Can you work these out from the model? Positions are in its coordinate system, mm. Give positions to 0.01 mm unless a question says otherwise; leave off trailing zeros. Use one line per item in the form item = value. Start each with the question number.
1) We'd pull the mould along X, two halves only. Please class faces 1 (the flat face through (0, 0, 12.326)), 2 (the cylindrical face through (-1.924, 0.028, -8.664)): released by +X, released by -X, zero draft, split by the parting line, or undercut.
2) Please list where these lines run through material, in increasing order: probe 1 along Z at (x, y) = (0, -1) (3 decimals); probe 2 along Z at (x, y) = (7.25, 1); probe 3 along Z at (x, y) = (-6.75, -0.5).
3) Suppose I cut it at A-A, the plane x = -5. State how many separate pieces and enclosed holes the cut face has, and give its area (3 significant figures).
4) For pin 1 (4 mm diameter, centred on x = -3.5, z = -7, fed in from +Y); pin 2 (1 mm diameter, centred on y = 0, z = 6, fed in from -X); pin 3 (10 mm diameter, centred on x = 6.5, z = -6.5, fed in from -Y), each with a flat end and sliding along its axis, tell me the tip position at first contact or that it passes through.
```python
from build123d import *

# Parameters (mm, degrees)
F0_R          = 8.875
F3_DEPTH      = 3
F3_DEPTH_BACK = 3
F4_SIZE       = 1


with BuildPart() as f2:
    # F0 (on Front) → F2 (revolve)
    with BuildSketch(Plane.XZ):
        with BuildLine():
            ThreePointArc((0, 10.375), (2.3580401671, 10.1034781917), (4.5926568488, 9.3031246401))
            ThreePointArc((4.5926568488, 9.3031246401), (7.0784745003, 10.5329995788), (9.1944970191, 12.325854972))
            Line((9.1944970191, 12.325854972), (0, 12.325854972))
            Line((0, 12.325854972), (0, 10.375))
        make_face()
    revolve(axis=Axis((0, 0, 0), (0, 0, 1)))

    # F0 (on Front) → F3 (join, two sides)
    with BuildSketch(Plane.XZ) as f3_sk:
        with BuildLine():
            ThreePointArc((0, 10.375), (-7.3362328548, -7.3362328548), (10.375, 0))
            ThreePointArc((10.375, 0), (8.8116241354, 5.4768517505), (4.5926568488, 9.3031246401))
            Line((4.5926568488, 9.3031246401), (0, 9.3031246401))
            Line((0, 9.3031246401), (0, 10.375))
        make_face()
        Circle(F0_R, mode=Mode.SUBTRACT)
        with BuildLine():
            Line((0, 9.3031246401), (4.5926568488, 9.3031246401))
            ThreePointArc((4.5926568488, 9.3031246401), (2.3580401671, 10.1034781917), (0, 10.375))
            Line((0, 10.375), (0, 9.3031246401))
        make_face()
    extrude(amount=F3_DEPTH)
    extrude(f3_sk.sketch, amount=-F3_DEPTH_BACK)

    # F4
    f4_edges = [f2.edges().sort_by_distance(p)[0] for p in [
        (-8.875, -3, 0),
        (-8.875, 3, 0),
    ]]
    chamfer(f4_edges, length=F4_SIZE)


solid = f2.part
```
Result sheet:
q1.face_1 = zero draft
q1.face_2 = undercut
q2.probe_1 = -10.375 to -8.875, 8.875 to 12.326
q2.probe_2 = -7.42 to -5.12, 5.12 to 7.42, 10.7 to 12.33
q2.probe_3 = -7.88 to -5.76, 5.76 to 7.88, 10.34 to 12.33
q3.separate_pieces = 3
q3.enclosed_holes = 0
q3.area = 49.4 mm²
q4.pin_1 = 2.95
q4.pin_2 = -8.8
q4.pin_3 = -3
